Read the model definition and answer for the solid it produces. Units are mm, in the model's axes. A direction names the side the tool comes from. Give positions to 0.01 mm unless a question says otherwise; leave off trailing zeros. Write each loop counter-clockwise with the first axis right and the second up, starting at its lowest first coordinate (ties: lowest second). Pieces come first, ordered by that corner, then holes. Notation, with made-up numbers: (-12.75, 48.25) - (23.25, 48.25) arc R33 cw to (23.25, 82.25) - close; hole circle Ø8 at (-6, -14). An arc over 180 degrees is marked (long way). Use CSV: the item, a comma, the result in double quotes. Start each with the question number.
from build123d import *

# Parameters (mm, degrees)
SKETCH1_W               = 40
SKETCH1_H               = 40
BOSS_EXTRUDE1_DEPTH     = 30
SKETCH2_R               = 4
CUT_EXTRUDE1_DEPTH      = 42.231056256
CUT_EXTRUDE2_DEPTH      = 54.851648071
CUT_EXTRUDE2_DEPTH_BACK = 54.851648071
SKETCH3_R               = 5
SKETCH4_W               = 10
SKETCH4_H               = 25
CUT_EXTRUDE3_DEPTH      = 54.851648071


with BuildPart() as part:
    # Sketch1 → Boss-Extrude1 (new body)
    with BuildSketch(Plane(origin=(0, 0, 0), x_dir=(1, 0, 0), z_dir=(0, 1, 0))):
        Rectangle(SKETCH1_W, SKETCH1_H)
    extrude(amount=BOSS_EXTRUDE1_DEPTH)

    # Sketch2 → Cut-Extrude1 (cut, through all)
    with BuildSketch(Plane(origin=(0, 30, 0), x_dir=(1, 0, 0), z_dir=(0, 1, 0))):
        with Locations(Location((0, 0, 0), (0, 0, 270))):
            Circle(SKETCH2_R)
    extrude(amount=-CUT_EXTRUDE1_DEPTH, mode=Mode.SUBTRACT)

    # Sketch3 → Cut-Extrude2 (cut, two sides: drawn at the far end of the back side and taken through both)
    with BuildSketch(Plane.ZY.offset(20).offset(-CUT_EXTRUDE2_DEPTH_BACK)):
        with Locations((12, 20)):
            Circle(SKETCH3_R)
    extrude(amount=CUT_EXTRUDE2_DEPTH + CUT_EXTRUDE2_DEPTH_BACK, mode=Mode.SUBTRACT)

    # Sketch4 → Cut-Extrude3 (cut, through all)
    with BuildSketch(Plane.ZY.offset(20)):
        with Locations((-15, 17.5)):
            Rectangle(SKETCH4_W, SKETCH4_H)
    extrude(amount=-CUT_EXTRUDE3_DEPTH, mode=Mode.SUBTRACT)


solid = part.part
(1) The part is cut by section A-A on y = 20. Write down the section's boundary in (x, z), plus the area to 3 significant figures.
(2) The part is cut by section D-D on x = 16.5. Write down the section's boundary in (y, z), plus the area to 3 significant figures.
(3) For a pull along Z with two mould halves and no side action, classify faces 1 (the face through (-3.905, 15.21, -0.867)), 2 (the face through (0.28, 15.564, 14.307)), 3 (the face through (0, 2, -20)), 4 (the face through (0, 5, -15)) as pulls with the +Z half, pulls with the -Z half, needs draft (parallel to the pull), parting line crosses it, or undercut.
(4) The part is cut by section C-C on z = 0. Write down the section's boundary in (x, y), plus the area to 3 significant figures.
(5) The part is cut by section B-B on x = 0. Write down the section's boundary in (y, z).
(6) Consider probe 1 along X at (y, z) = (19.25, 0); probe 2 along Y at (x, z) = (-5, 12); probe 3 along Z at (x, y) = (-9.5, 20). Determine where each line is inside the solid, lowest interval first.
(7) Which of the six approach directions +Z, -Z, +X, -X, +Y, -Y give full straight-line access (tool end or side, diameter ignored) to faces 5 (the face through (0, 17, -10)), 6 (the face through (0, 30, 5))?
(8) Given P1, Ø3, axis at x = 11.5, y = 19, coming from the -Z side; P2, Ø1, axis at x = 13, z = -13, coming from the +Y side, each flat-ended and moving along its own axis, determine where each tip first touches the part or whether it passes through.
Reported:
1,outline,"(-20, -10) - (20, -10) - (20, 7) - (-20, 7) - close; (-20, 17) - (20, 17) - (20, 20) - (-20, 20) - close; hole circle Ø8 at (0, 0)"
1,area,"750 mm²"
2,outline,"(0, -20) - (5, -20) - (5, -10) - (30, -10) - (30, 20) - (0, 20) - close; hole circle Ø10 at (20, 12)"
2,area,"871 mm²"
3,face 1,"undercut"
3,face 2,"undercut"
3,face 3,"pulls with the -Z half"
3,face 4,"needs draft"
4,outline,"(-20, 0) - (-4, 0) - (-4, 30) - (-20, 30) - close; (4, 0) - (20, 0) - (20, 30) - (4, 30) - close"
4,area,"960 mm²"
5,outline,"(0, -20) - (5, -20) - (5, -10) - (30, -10) - (30, -4) - (0, -4) - close; (0, 4) - (30, 4) - (30, 20) - (0, 20) - close; hole circle Ø10 at (20, 12)"
6,probe 1,"-20 to -4, 4 to 20"
6,probe 2,"0 to 15, 25 to 30"
6,probe 3,"-10 to 7, 17 to 20"
7,face 5,"-Z, +X, -X, +Y"
7,face 6,"+Z, -Z, +X, -X, +Y"
8,P1,"z = -10"
8,P2,"y = 5"
